Autodesk Inventor part; units mm, degrees
ref_plane "YZ Plane" through (0, 0, 0) normal (1, 0, 0) x (0, 1, 0)
ref_plane "XZ Plane" through (0, 0, 0) normal (0, 1, 0) x (-1, 0, 0)
ref_plane "XY Plane" through (0, 0, 0) normal (0, 0, 1) x (1, 0, 0)
sketch "Sketch2" plane through (0, 0, 0) normal (0, 0, 1) x (1, 0, 0)
  circle A0 centre (46.408, 50.5954) radius 3.175 construction
  circle A1 centre (46.408, 50.5954) radius 5.08
  line L0 (46.408, 50.5954) -> (38.8405, 52.8571) construction
  line L1 (46.408, 50.5954) -> (53.477, 47.0722) construction
  circle A2 centre (38.8405, 52.8571) radius 2.8183
  circle A3 centre (53.477, 47.0722) radius 2.8183
  circle A4 centre (38.8405, 52.8571) radius 1.25
  circle A5 centre (53.477, 47.0722) radius 1.25
  line L2 (38.8405, 55.6754) -> (46.408, 55.6754)
  line L3 (37.5063, 50.3746) -> (42.0976, 47.9072)
  line L4 (55.4024, 49.1303) -> (50.0414, 54.1458)
  line L5 (52.3888, 44.4725) -> (48.6507, 46.0372)
  circle A6 centre (46.408, 50.5954) radius 3
  circle A7 centre (46.408, 50.5954) radius 4.2333 construction
  line L6 (46.408, 50.5954) -> (42.9902, 43.4749) construction
  circle A8 centre (42.9902, 43.4749) radius 1.25
  circle A9 centre (42.9902, 43.4749) radius 2.8183
  line L7 (40.2199, 43.993) -> (41.3557, 50.0663)
  line L8 (45.2023, 41.7287) -> (48.5744, 46.0005)
  point P0 (0, 0)
  dimension "d7" = 10.16
  dimension "d8" = 2.5
  dimension "d9" = 6
  dimension "d10" = 8.4667
extrude "Plate2" add sketch "Sketch2" along normal blind 4 contours A1 | A3 | A1 A2 L2 | A1 L7 L3 A2 | A2 | A1 L3 L7 | A9
sketch "Sketch3" plane through (0, 0, 4) normal (0, 0, 1) x (1, 0, 0)
  arc A0 (42.0976, 47.9072) -> (44.2097, 46.0157) centre (46.408, 50.5954) ccw
  circle A1 centre (46.408, 50.5954) radius 5.08
  circle A2 centre (42.9902, 43.4749) radius 2.8183
  line L0 (40.2108, 43.9416) -> (41.328, 50.5954)
  line L1 (45.1528, 41.6677) -> (48.9266, 46.1837)
  arc A3 (44.2097, 46.0157) -> (50.9546, 48.3294) centre (46.408, 50.5954) ccw
  point P0 (0, 0)
sheet face with bend "Face3" sketch "Sketch3" thickness 4 toward (0, 0, -1) bend radius 4 contours A0 A2 L0 A1 | A1 L1 A2
bend "Bend1"
sketch "Sketch4" plane through (0, 0, 4) normal (0, 0, 1) x (1, 0, 0)
  arc A0 (50.9546, 48.3294) -> (46.408, 55.6754) centre (46.408, 50.5954) ccw
  arc A1 (50.9546, 48.3294) -> (46.408, 55.6754) centre (46.408, 50.5954) ccw
  circle A2 centre (46.408, 50.5954) radius 5.08
  circle A3 centre (53.477, 47.0722) radius 2.8183
  line L0 (55.4038, 49.129) -> (49.8811, 54.3027)
  line L1 (52.9948, 44.2955) -> (45.5388, 45.5903)
  arc A4 (44.2097, 46.0157) -> (50.9546, 48.3294) centre (46.408, 50.5954) ccw
  line L2 (49.8811, 54.3027) -> (45.5388, 45.5903)
  point P0 (0, 0)
sheet face with bend "Face4" sketch "Sketch4" thickness 4 toward (0, 0, -1) bend radius 4 picked at (48.6605, 51.1377) contours A2 L2 A0 | A3 L1 A2 | A0 L0 A3
bend "Bend2"
sketch "Sketch5" plane through (0, 0, 4) normal (0, 0, 1) x (1, 0, 0)
  arc A0 (48.8803, 52.2948) -> (46.5396, 47.5983) centre (46.408, 50.5954) ccw
  arc A1 (48.8803, 52.2948) -> (46.5396, 47.5983) centre (46.408, 50.5954) ccw
  circle A2 centre (46.408, 50.5954) radius 3
  point P0 (0, 0)
  point P1 (46.5396, 47.5983)
extrude "Extrusion1" cut sketch "Sketch5" against normal blind 25.4
fillet "Fillet1" radius 3.175 2 edges at (40.9777, 48.509, 2) (48.0642, 45.1518, 2)
sketch "Sketch6" plane through (0, 0, 4) normal (0, 0, 1) x (1, 0, 0)
  circle A0 centre (46.408, 50.5954) radius 3
  line L0 (43.408, 53.5954) -> (49.408, 53.5954)
  line L1 (49.408, 53.5954) -> (49.408, 47.5954)
  line L2 (49.408, 47.5954) -> (43.408, 47.5954)
  line L3 (43.408, 47.5954) -> (43.408, 53.5954)
  line L4 (43.408, 52.9954) -> (49.408, 52.9954)
  point P0 (0, 0)
  point P1 (44.608, 52.9954)
  point P2 (48.208, 52.9954)
  dimension "d26" = 5.4
extrude "Extrusion2" add sketch "Sketch6" against normal up to surface (4 mm away) contours L4 A0 picked at (46.6209, 53.1725)
equation "\"d12\" = Thickness"
equation "\"d13\" = BendRadius"
equation "\"d14\" = BendReliefWidth"
equation "\"d16\" = MinimumRemnant"
equation "\"d15\" = BendReliefDepth"
equation "\"d17\" = TransitionRadius"
equation "\"d18\" = BendRadius"
equation "\"d19\" = BendReliefWidth"
equation "\"d21\" = MinimumRemnant"
equation "\"d20\" = BendReliefDepth"
equation "\"d22\" = TransitionRadius"
equation "\"BendRadius\" = Thickness"
equation "\"BendReliefWidth\" = Thickness"
equation "\"BendReliefDepth\" = 0.5 * Thickness"
equation "\"CornerReliefSize\" = 4 * Thickness"
equation "\"MinimumRemnant\" = 2 * Thickness"
equation "\"TransitionRadius\" = BendRadius"
equation "\"JacobiRadiusSize\" = BendRadius"
equation "\"GapSize\" = Thickness"
properties part number "ShaftLock"
Work out the finished part from the listing and answer in its coordinate system (mm). A direction names the side the tool comes from. Round coordinates to 2 decimals unless told otherwise and drop trailing zeros. Loops run counter-clockwise (first coordinate to the right, second up) from the corner with the lowest first, then second, coordinate; pieces in that order, holes last. Notation, with made-up numbers: M 3.5,56.5 L 12.5,56.5 A29 ccw 12.5,95.5 Z; hole C -35,41.5 d5. An arc over 180 degrees is marked long. Use CSV: the item, a comma, the result in double quotes.
Q1. A tool of negligible diameter and unlimited length cuts with its end or side. For faces 4 (the flat face through (40.403, 45.087, 2.028)), 5 (the flat face through (46, 52.995, 2)), 6 (the flat face through (51.454, 44.563, 2.028)), from which of +Z, -Z, +X, -X, +Y, -Y can it reach the whole face along a straight path? Write none if from no direction.
Determined:
face 4,"+Z, -Z, -X"
face 5,"+Z, -Z"
face 6,"+Z, -Z, -Y"
Q2. The mould has two halves that part along X. Classify faces 1 (the flat face through (43, 55.675, 2)), 2 (the cylindrical face through (48.255, 44.699, 2.028)), 3 (the cylindrical face through (36.095, 53.494, 1.972)): pulls with the +X half, pulls with the -X half, needs draft (parallel to the pull), parting line crosses it, or undercut.
Determined:
face 1,"needs draft"
face 2,"undercut"
face 3,"pulls with the -X half"
Q3. Section C-C, the plane z = 1 is taken. State how many separate pieces and enclosed holes the cut face has, then the cut area to 3 significant figures.
Determined:
separate pieces,"1"
enclosed holes,"4"
area,"147 mm2"
Q4. Section A-A, the plane y = 48 is taken. Determine the outline of the cut face in (x, z), then the cut area to 3 significant figures.
Determined:
outline,"M 40.4,0 L 44.9,0 L 44.9,4 L 40.4,4 Z; M 47.91,0 L 52.64,0 L 52.64,4 L 47.91,4 Z; M 54.31,0 L 56.14,0 L 56.14,4 L 54.31,4 Z"
area,"44.2 mm2"
Q5. Section D-D, the plane y = 51.25 is taken. Determine the outline of the cut face in (x, z), then the cut area to 3 significant figures.
Determined:
outline,"M 36.53,0 L 43.48,0 L 43.48,4 L 36.53,4 Z; M 49.34,0 L 53.14,0 L 53.14,4 L 49.34,4 Z"
area,"43.0 mm2"
Q6. Consider L1, parallel to Y at x = 43.75, z = 0.4; L2, parallel to Y at x = 46.75, z = 3.45; L3, parallel to X at y = 50.75, z = 2.6. Determine where each line is inside the solid, lowest interval first.
Determined:
L1,"40.76 to 42.48, 44.47 to 49.2, 51.99 to 55.68"
L2,"43.58 to 47.61, 53 to 55.66"
L3,"36.97 to 43.41, 49.4 to 53.67"
Q7. Section B-B, the plane x = 53.5 is taken. Determine the outline of the cut face in (y, z), then the cut area to 3 significant figures.
Determined:
outline,"M 44.25,0 L 45.82,0 L 45.82,4 L 44.25,4 Z; M 48.32,0 L 50.91,0 L 50.91,4 L 48.32,4 Z"
area,"16.6 mm2"
